Can you work these out from the model? Positions are in its coordinate system, mm. Face numbers are marked on the shaded views. A direction names the side the tool comes from. Round coordinates to 2 decimals unless told otherwise and drop trailing zeros. Write each loop counter-clockwise with the first axis right and the second up, starting at its lowest first coordinate (ties: lowest second). Pieces come first, ordered by that corner, then holes. Notation, with made-up numbers: (35, 25.5) -> (82, 25.5) arc R12 ccw to (82, 36.5) -> close; hole circle Ø7 at (37, 70). An arc over 180 degrees is marked (long way). Use CSV: the item, a comma, the result in double quotes.
```python
from build123d import *

# Parameters (mm, degrees)
SKETCH1_W           = 300
SKETCH1_H           = 100
BOSS_EXTRUDE1_DEPTH = 80
SHELL1_T            = -5
SKETCH2_W           = 12
SKETCH2_H           = 23
BOSS_EXTRUDE2_DEPTH = 1
SKETCH3_W           = 8
SKETCH3_H           = 19
BOSS_EXTRUDE3_DEPTH = 5
BOSS_EXTRUDE4_DEPTH = 8
SKETCH6_R           = 0.5


with BuildPart() as part:
    # Sketch1 → Boss-Extrude1 (new body)
    with BuildSketch(Plane(origin=(0, 0, 0), x_dir=(1, 0, 0), z_dir=(0, 1, 0))):
        Rectangle(SKETCH1_W, SKETCH1_H)
    extrude(amount=BOSS_EXTRUDE1_DEPTH)

    # Shell1
    shell1_openings = [part.faces().sort_by_distance(p)[0] for p in [
        (0, 80, 0),
    ]]
    offset(amount=SHELL1_T, openings=shell1_openings, kind=Kind.INTERSECTION)

    # Sketch2 → Boss-Extrude2 (add)
    with BuildSketch(Plane.XY.offset(50)):
        with Locations((0, 63.5)):
            Rectangle(SKETCH2_W, SKETCH2_H)
    extrude(amount=BOSS_EXTRUDE2_DEPTH)

    # Sketch3 → Boss-Extrude3 (add)
    with BuildSketch(Plane.XY.offset(51)):
        with Locations((0, 63.5)):
            Rectangle(SKETCH3_W, SKETCH3_H)
    extrude(amount=BOSS_EXTRUDE3_DEPTH)

    # Sketch4 → Boss-Extrude4 (add)
    with BuildSketch(Plane(origin=(4, 0, 0), x_dir=(0, 0, -1), z_dir=(1, 0, 0))):
        with BuildLine():
            Line((-56, 54), (-53.5, 54))
            ThreePointArc((-53.5, 54), (-55.03079013, 51.083775539), (-57.395060139, 48.790762051))
            ThreePointArc((-57.395060139, 48.790762051), (-56.354803681, 51.303597174), (-56, 54))
        make_face()
    extrude(amount=-BOSS_EXTRUDE4_DEPTH)

    # Sweep1: sweep along a path in Sketch5
    with BuildLine(Plane.XY.offset(53)) as sweep1_path:
        Line((-4, 63.5), (-7, 63.5))
        ThreePointArc((-7, 63.5), (-8.414213562, 62.914213562), (-9, 61.5))
        Line((-9, 61.5), (-9, 41.5))
        ThreePointArc((-9, 41.5), (-8.414213562, 40.085786438), (-7, 39.5))
        Line((-7, 39.5), (7, 39.5))
        ThreePointArc((7, 39.5), (8.414213562, 40.085786438), (9, 41.5))
        Line((9, 41.5), (9, 61.5))
        ThreePointArc((9, 61.5), (8.414213562, 62.914213562), (7, 63.5))
        Line((7, 63.5), (4, 63.5))
    # Sketch6 → Sweep1 (sweep)
    with BuildSketch(Plane.ZY.offset(4)):
        with Locations((53, 63.5)):
            Circle(SKETCH6_R)
    sweep(path=sweep1_path.line)


solid = part.part
```
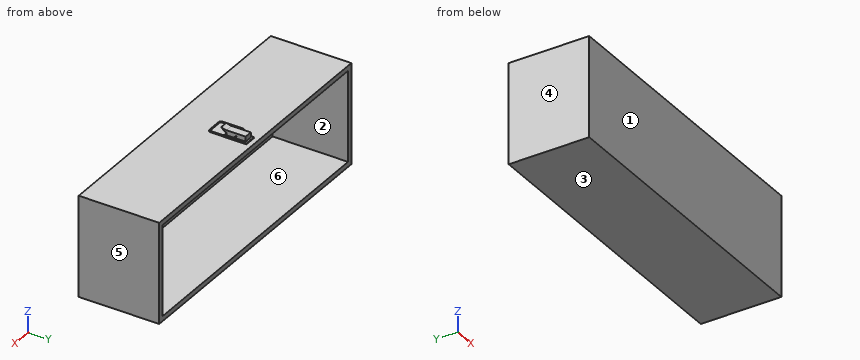
Q1. If we mould it in two halves opening along X, with no side actions, what happens to the marked faces 3, 4, 5 and 6? For each: released by +X, released by -X, zero draft, split by the parting line, or undercut.
Resolved:
face 3,"zero draft"
face 4,"released by -X"
face 5,"released by +X"
face 6,"undercut"
Q2. Suppose I cut it at C-C (x = -57). Write out the boundary of the cut face in (y, z), and give its area (3 significant figures).
Resolved:
outline,"(0, -50) -> (80, -50) -> (80, -45) -> (5, -45) -> (5, 45) -> (80, 45) -> (80, 50) -> (0, 50) -> close"
area,"1,250 mm^2"
Q3. Suppose I cut it at A-A (y = 30.5). Write out the boundary of the cut face in (x, z).
Resolved:
outline,"(-150, -50) -> (150, -50) -> (150, 50) -> (-150, 50) -> close; hole (-145, -45) -> (145, -45) -> (145, 45) -> (-145, 45) -> close"
Q4. Suppose I cut it at B-B (z = -16.5). Write out the boundary of the cut face in (x, y).
Resolved:
outline,"(-150, 0) -> (150, 0) -> (150, 80) -> (145, 80) -> (145, 5) -> (-145, 5) -> (-145, 80) -> (-150, 80) -> close"
Q5. On a 3-axis mill with a long thin cutter (end or side, diameter ignored), from which of +Z, -Z, +X, -X, +Y, -Y can I reach the whole of each face in a straight line? I mean the marked faces 1 and 2. Say none if no direction works.
Resolved:
face 1,"+Z, -Z, +X, -X, -Y"
face 2,"+Y"
Q6. Please list where these lines run through material, in increasing order: probe 1 along X at (y, z) = (55.5, 2.5); probe 2 along Z at (x, y) = (116.5, 35); probe 3 along Y at (x, z) = (-21.5, -18).
Resolved:
probe 1,"x = -150 to -145, 145 to 150"
probe 2,"z = -50 to -45, 45 to 50"
probe 3,"y = 0 to 5"
Q7. Will these pins go through, and if not, where does the flat tip stop? P1, Ø5, axis at x = -25.5, y = 49, coming from the +Z side; P2, Ø9.5, axis at x = -1, y = 61, coming from the +Z side; P3, Ø0.8, axis at x = -0.5, z = 50.5, coming from the +Y side.
Resolved:
P1,"stops at z = 50"
P2,"stops at z = 56"
P3,"stops at y = 75"
